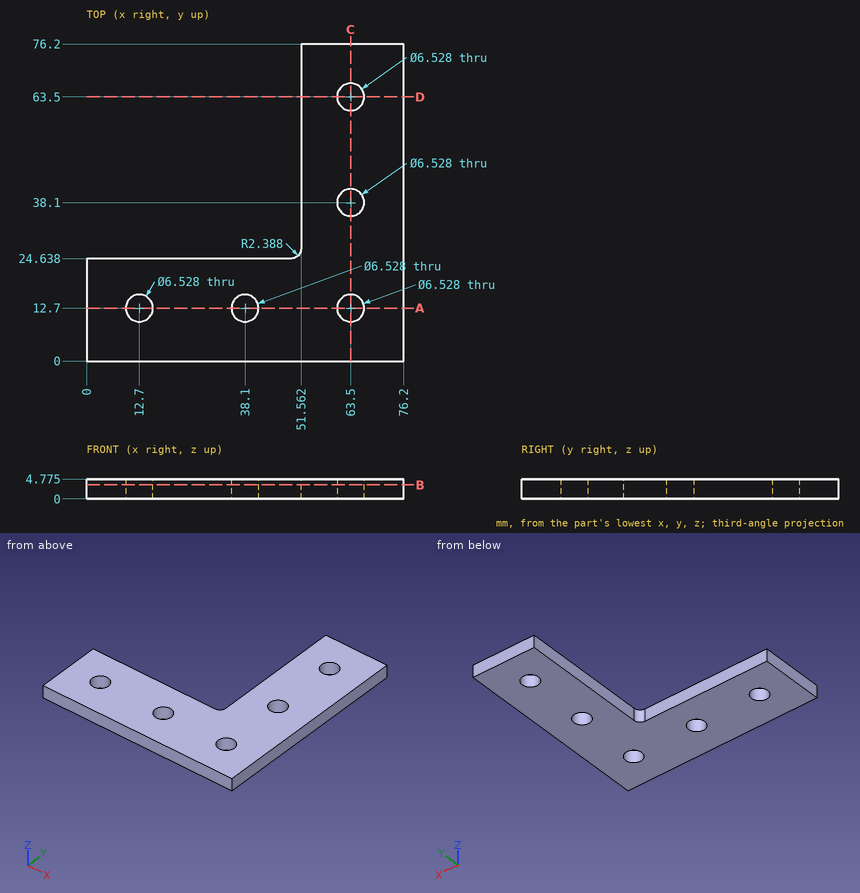
Can you work these out from the drawing? Everything is in mm from the part's minimum corner. Give positions to 0.01 mm unless a question says otherwise; leave off trailing zeros. Order: outer loops, then holes, each group sorted by start corner. A loop starts at its lowest first (then second) coordinate and runs counter-clockwise, first axis right, second up. Notation, with made-up numbers: M -29.75,89 L 2.25,89 A20 cw 2.25,104 Z; hole C 2.5,70.25 d2. An arc over 180 degrees is marked long. One line per item, written item: value.
Item 1: If we section it at D-D on y = 63.5: Write out the boundary of the cut face in (x, z) (1 decimal).
Verdict:
outline: M 51.6,0 L 60.2,0 L 60.2,4.8 L 51.6,4.8 Z; M 66.8,0 L 76.2,0 L 76.2,4.8 L 66.8,4.8 Z
Item 2: If we section it at A-A on y = 12.7: Write out the boundary of the cut face in (x, z) (1 decimal).
Verdict:
outline: M 0,0 L 9.4,0 L 9.4,4.8 L 0,4.8 Z; M 16,0 L 34.8,0 L 34.8,4.8 L 16,4.8 Z; M 41.4,0 L 60.2,0 L 60.2,4.8 L 41.4,4.8 Z; M 66.8,0 L 76.2,0 L 76.2,4.8 L 66.8,4.8 Z
Item 3: If we section it at B-B on z = 3.35: Write out the boundary of the cut face in (x, y) (1 decimal), and give its area (3 significant figures).
Verdict:
outline: M 0,0 L 76.2,0 L 76.2,76.2 L 51.6,76.2 L 51.6,27 A2.4 cw 49.2,24.6 L 0,24.6 Z; hole C 12.7,12.7 d6.5; hole C 38.1,12.7 d6.5; hole C 63.5,12.7 d6.5; hole C 63.5,38.1 d6.5; hole C 63.5,63.5 d6.5
area: 2,980 mm2
Item 4: For pin 1 (5 mm diameter, centred on x = 63.5, y = 63.5, fed in from -Z); pin 2 (1.4 mm diameter, centred on y = 43, z = 1.5, fed in from -X), each with a flat end and sliding along its axis, tell me the tip position at first contact or that it passes through.
Verdict:
pin 1: through
pin 2: x = 51.56
Item 5: Please list where these lines run through material, in increasing order: line 1 (X direction, y = 38, z = 1.85); line 2 (Y direction, x = 4.5, z = 3); line 3 (X direction, y = 43, z = 2.7).
Verdict:
line 1: 51.56 to 60.24, 66.76 to 76.2
line 2: 0 to 24.64
line 3: 51.56 to 76.2
